Geometry: final body of the model. Coordinates: model frame, mm. A direction names the side the tool comes from. Round coordinates to 2 decimals unless told otherwise and drop trailing zeros. Loops run counter-clockwise (first coordinate to the right, second up) from the corner with the lowest first, then second, coordinate; pieces in that order, holes last. Notation, with made-up numbers: (-29, 19) - (17, 19) arc R13 ccw to (17, 29) - close; hole circle Ø11 at (35, -2). An arc over 180 degrees is marked (long way). Answer as a JSON object with one key per item and string values. Group by question number.
Item 1: First-contact query: pin 1 (2.5 mm diameter, centred on y = -9.5, z = -9, fed in from -X); pin 2 (6 mm diameter, centred on x = -7.5, y = -0.5, fed in from -Z); pin 3 (8 mm diameter, centred on x = -6, z = -10.5, fed in from -Y). Flat tips, straight axial feed; report the tip coordinate or a pass-through.
Item 2: Section D-D (z = 28). Return the cut outline in (x, y), plus the area to 3 significant figures.
Item 3: Reachability of faces 1 (the face through (-24, -0.4, -2)), 2 (the face through (-26.2, 0, 17)), 3 (the face through (0, 9, 11)) from +Z, -Z, +X, -X, +Y, -Y: full face, straight path, thin tool, end or side. Return the list, or none.
Item 4: Line query: line 1 (Y direction, x = -3, z = -4.5); line 2 (X direction, y = 11.5, z = 11); line 3 (Y direction, x = 5.6, z = 0). Output: solid intervals per line, ascending.
Item 5: Section A-A (x = -3.5). Count the separate pieces of the cut face and the enclosed holes in it, plus the area to 3 significant figures.
Item 6: Section B-B (y = -13.5). Return the cut outline in (x, z).
Item 7: Draft query along Z for faces 4 (the face through (-8, 0, 11)), 5 (the face through (-24, 10, 5)), 6 (the face through (0.34, 0.02, -7.25)). Return one class per face: released by +Z, released by -Z, zero draft, split by the parting line, or undercut.
Item 8: Section C-C (x = -7). Return the cut outline in (y, z), plus the area to 3 significant figures.
Autodesk Inventor part; units mm, degrees
ref_plane "verschluss_XY" through (-1, 0, 0) normal (1, 0, 0) x (0, 0, -1)
ref_plane "verschluss_YZ" through (-1, 0, 0) normal (0, 0, -1) x (0, 1, 0)
ref_plane "verschluss_ZX" through (-1, 0, 0) normal (0, 1, 0) x (1, 0, 0)
sketch "Sketch_1" plane through (0, 0, 0) normal (0, 1, 0) x (-1, 0, 0)
  line L0 (0, 16) -> (-2, 16)
  line L1 (-2, 16) -> (-6, 12)
  line L2 (-6, 12) -> (-6, -20)
  line L3 (-6, -20) -> (-4, -20)
  line L4 (-4, -20) -> (0, -16)
  line L5 (0, -16) -> (0, 16)
extrude "Extrusion1" add sketch "Sketch_1" along normal mid plane 32
sketch "Sketch_2" plane through (0, 0, 0) normal (1, 0, 0) x (0, 1, 0)
  line L0 (15, 15) -> (-15, 15)
  line L1 (-15, 15) -> (-15, -15)
  line L2 (-15, -15) -> (15, -15)
  line L3 (15, -15) -> (15, 15)
extrude "Extrusion2" add sketch "Sketch_2" against normal blind 1
sketch "Sketch_3" plane through (0, 0, 0) normal (1, 0, 0) x (0, 1, 0)
  line L0 (11, 11) -> (-11, 11)
  line L1 (-11, 11) -> (-11, -11)
  line L2 (-11, -11) -> (11, -11)
  line L3 (11, -11) -> (11, 11)
extrude "Extrusion3" cut sketch "Sketch_3" along normal mid plane 3
sketch "Sketch_5" plane through (0, 0, 0) normal (0, 1, 0) x (-1, 0, 0)
  line L0 (15, -9) -> (15, 9)
  line L1 (15, 9) -> (-1.5, 9)
  line L2 (-1.5, 9) -> (-1.5, -9)
  line L3 (-1.5, -9) -> (15, -9)
extrude "Extrusion4" add sketch "Sketch_5" along normal mid plane 18
sketch "Sketch_4" plane through (0, 0, 0) normal (0, 1, 0) x (-1, 0, 0)
  line L0 (15, -6) -> (15, 6)
  line L1 (15, 6) -> (-1.5, 6)
  line L2 (-1.5, 6) -> (-1.5, -6)
  line L3 (-1.5, -6) -> (15, -6)
extrude "Extrusion5" add sketch "Sketch_4" along normal mid plane 22
sketch "Sketch_7" plane through (0, 0, 0) normal (0, 0, 1) x (1, 0, 0)
  line L0 (-15, 6) -> (-15, -6)
  line L1 (-15, -6) -> (1.5, -6)
  line L2 (1.5, -6) -> (1.5, 6)
  line L3 (1.5, 6) -> (-15, 6)
extrude "Extrusion6" add sketch "Sketch_7" along normal mid plane 22
sketch "Sketch_10" plane through (0, 0, 0) normal (0, 0, 1) x (1, 0, 0)
  line L0 (-15, 0) -> (-20.45, 0)
  line L1 (-20.45, 0) -> (-26.2, 5.75)
  line L2 (-26.2, 5.75) -> (-26.2, 10)
  line L3 (-26.2, 10) -> (-17.2, 10)
  line L4 (-17.2, 10) -> (-16.2, 9)
  line L5 (-16.2, 9) -> (-16.2, 5)
  line L6 (-16.2, 5) -> (-15, 5)
  line L7 (-15, 5) -> (-15, 0)
  line L8 (-15, 0) -> (-20.45, 0)
revolve "Revolution1" add sketch "Sketch_10" angle 360 about axis through (-15, 0, 0) along (1, 0, 0)
sketch "Sketch_11" plane through (0, 0, 0) normal (0, 0, 1) x (1, 0, 0)
  line L0 (-20.4, 0) -> (-26.2, 0)
  line L1 (-25.7, 0) -> (-25.7, 4.65)
  line L2 (-25.7, 4.65) -> (-25.05, 4.65)
  line L3 (-25.05, 4.65) -> (-20.4, 0)
  line L4 (-20.4, 0) -> (-25.7, 0)
revolve "Revolution2" add sketch "Sketch_11" angle 360 about axis through (-20.4, 0, 0) along (1, 0, 0)
sketch "Sketch_12" plane through (-25.7, 0, 0) normal (1, 0, 0) x (0, 0, -1)
  line L0 (-2.65, 0.4) -> (-2.65, -0.4)
  line L1 (-2.65, -0.4) -> (-0.4, -0.4)
  line L2 (-0.4, -0.4) -> (-0.4, -2.65)
  line L3 (-0.4, -2.65) -> (0.4, -2.65)
  line L4 (0.4, -2.65) -> (0.4, -0.4)
  line L5 (0.4, -0.4) -> (2.65, -0.4)
  line L6 (2.65, -0.4) -> (2.65, 0.4)
  line L7 (2.65, 0.4) -> (0.4, 0.4)
  line L8 (0.4, 0.4) -> (0.4, 2.65)
  line L9 (0.4, 2.65) -> (-0.4, 2.65)
  line L10 (-0.4, 2.65) -> (-0.4, 0.4)
  line L11 (-0.4, 0.4) -> (-2.65, 0.4)
extrude "Extrusion7" cut sketch "Sketch_12" along normal blind 3
sketch "Sketch_13" plane through (-26.2, 0, 0) normal (1, 0, 0) x (0, 0, -1)
  arc A0 (-44, -5) -> (-39, -10) centre (-39, -5) ccw
  line L0 (-39, -10) -> (-16, -10)
  arc A1 (-12, -12) -> (-16, -10) centre (-16, -15) ccw
  line L1 (-12, -12) -> (-9.2, -12)
  line L2 (-9.2, -12) -> (-9.2, -10)
  line L3 (-9.2, -10) -> (0, -10)
  line L4 (0, -10) -> (0, -6)
  arc A2 (0, 6) -> (0, -6) centre (0, 0) ccw
  line L5 (0, 6) -> (0, 10)
  line L6 (0, 10) -> (-9.2, 10)
  line L7 (-9.2, 10) -> (-9.2, 12)
  line L8 (-9.2, 12) -> (-12, 12)
  arc A3 (-16, 10) -> (-12, 12) centre (-16, 15) ccw
  line L9 (-16, 10) -> (-39, 10)
  arc A4 (-39, 10) -> (-44, 5) centre (-39, 5) ccw
  line L10 (-44, 5) -> (-44, -5)
extrude "Extrusion8" add sketch "Sketch_13" along normal blind 4.3
sketch "Sketch_14" plane through (0, 0, 0) normal (0, 1, 0) x (-1, 0, 0)
  line L0 (28, 34) -> (28, 49)
  line L1 (28, 49) -> (18, 49)
  line L2 (18, 49) -> (18, 34)
  line L3 (18, 34) -> (21.9, 34)
  line L4 (21.9, 34) -> (21.9, 38.5431)
  arc A0 (23.0716, 41.3716) -> (21.9, 38.5431) centre (25.9, 38.5431) ccw
  line L5 (23.0716, 41.3716) -> (25.7, 44)
  line L6 (25.7, 44) -> (26.2, 44)
  line L7 (26.2, 44) -> (26.2, 34)
  line L8 (26.2, 34) -> (28, 34)
extrude "Extrusion9" cut sketch "Sketch_14" along normal mid plane 20
sketch "Sketch_15" plane through (-4.2, 0, 0) normal (1, 0, 0) x (0, 0, -1)
  circle A0 centre (0, 0) radius 8
extrude "Extrusion10" cut sketch "Sketch_15" along normal blind 10.2
sketch "Sketch_16" plane through (-4.2, 0, 0) normal (1, 0, 0) x (0, 0, -1)
  circle A0 centre (0, 0) radius 8
  arc A1 (-7.0931, 1.5) -> (-7.0931, -1.5) centre (0, 0) ccw
  line L0 (-7.0931, -1.5) -> (-4.4542, -1.5)
  arc A2 (-4.4542, -1.5) -> (4.4542, -1.5) centre (0, 0) ccw
  line L1 (4.4542, -1.5) -> (7.0931, -1.5)
  arc A3 (7.0931, -1.5) -> (7.0931, 1.5) centre (0, 0) ccw
  line L2 (7.0931, 1.5) -> (4.4542, 1.5)
  arc A4 (4.4542, 1.5) -> (-4.4542, 1.5) centre (0, 0) ccw
  line L3 (-4.4542, 1.5) -> (-7.0931, 1.5)
extrude "Extrusion11" add sketch "Sketch_16" along normal blind 9.2
sketch "Sketch_17" plane through (0, 0, 0) normal (1, 0, 0) x (0, 1, 0)
  circle A0 centre (0, 0) radius 1.5
extrude "Extrusion12" add sketch "Sketch_17" along normal mid plane 10
ref_plane "verschluss_XY" through (-1, 0, 0) normal (1, 0, 0) x (0, 0, -1)
ref_plane "verschluss_YZ" through (-1, 0, 0) normal (0, 0, -1) x (0, 1, 0)
ref_plane "verschluss_ZX" through (-1, 0, 0) normal (0, 1, 0) x (1, 0, 0)
properties part number "1XXX_01_05_1"
Values:
{
 "1": {"pin 1": "stops at x = -15", "pin 2": "stops at z = -11", "pin 3": "stops at y = -9"},
 "2": {"outline": "(-26.2, -10) - (-21.9, -10) - (-21.9, 10) - (-26.2, 10) - close", "area": "86.0 mm^2"},
 "3": {"face 1": "-X", "face 2": "+Z, -Z, -X, +Y, -Y", "face 3": "none"},
 "4": {"line 1": "y = -11 to -1.5, 1.5 to 11", "line 2": "x = -26.2 to -21.9, -1 to 6", "line 3": "y = -16 to -8, 8 to 16"},
 "5": {"separate pieces": "2", "enclosed holes": "1", "area": "342 mm^2"},
 "6": {"outline": "(-1, -15) - (0, -15) - (0, -16) - (4, -20) - (6, -20) - (6, 12) - (2, 16) - (0, 16) - (0, 15) - (-1, 15) - close"},
 "7": {"face 4": "released by +Z", "face 5": "zero draft", "face 6": "undercut"},
 "8": {"outline": "(-11, -6) - (-9, -6) - (-9, -9) - (-6, -9) - (-6, -11) - (6, -11) - (6, -9) - (9, -9) - (9, -6) - (11, -6) - (11, 6) - (9, 6) - (9, 9) - (6, 9) - (6, 11) - (-6, 11) - (-6, 9) - (-9, 9) - (-9, 6) - (-11, 6) - close", "area": "420 mm^2"}
}
